```python
from build123d import *

# Parameters (mm, degrees)
BOSS_EXTRUDE2_DEPTH = 40
SKETCH3_4_R         = 2
SKETCH3_4_R_2       = 1
BOSS_EXTRUDE3_DEPTH = 10
BOSS_EXTRUDE4_START = -20
SKETCH3_5_R         = 2
SKETCH3_5_R_2       = 1
BOSS_EXTRUDE4_DEPTH = 10
SKETCH5_R           = 2
CUT_EXTRUDE1_DEPTH  = 10
FILLET1_R           = 3
FILLET2_R           = 3


with BuildPart() as part:
    # Sketch3 → Boss-Extrude2 (new body)
    with BuildSketch(Plane.XY):
        with BuildLine():
            Line((14.107916892, 0), (14.107916892, 1))
            Line((14.107916892, 1), (-5.892083108, 1))
            ThreePointArc((-5.892083108, 1), (-5.863018057, 0.804975408), (-5.853298215, 0.608036602))
            ThreePointArc((-5.853298215, 0.608036602), (-5.877106832, 0.300355571), (-5.947965831, 0))
            Line((-5.947965831, 0), (14.107916892, 0))
        make_face()
    extrude(amount=-BOSS_EXTRUDE2_DEPTH)

    # Sketch3_4 → Boss-Extrude3 (add)
    with BuildSketch(Plane.XY):
        with Locations((-7.853298215, 0.608036602)):
            Circle(SKETCH3_4_R)
        with Locations((-7.853298215, 0.608036602)):
            Circle(SKETCH3_4_R_2, mode=Mode.SUBTRACT)
    extrude(amount=-BOSS_EXTRUDE3_DEPTH)

    # Sketch3_5 → Boss-Extrude4 (add)
    with BuildSketch(Plane.XY.offset(BOSS_EXTRUDE4_START)):
        with Locations((-7.853298215, 0.608036602)):
            Circle(SKETCH3_5_R)
        with Locations((-7.853298215, 0.608036602)):
            Circle(SKETCH3_5_R_2, mode=Mode.SUBTRACT)
    extrude(amount=-BOSS_EXTRUDE4_DEPTH)

    # Sketch5 → Cut-Extrude1 (cut)
    with BuildSketch(Plane(origin=(0, 1, 0), x_dir=(1, 0, 0), z_dir=(0, 1, 0))):
        with Locations((-0.892083108, 30)):
            Circle(SKETCH5_R)
        with Locations((-0.892083108, 10)):
            Circle(SKETCH5_R)
        with Locations((9.107916892, 20)):
            Circle(SKETCH5_R)
    extrude(amount=-CUT_EXTRUDE1_DEPTH, mode=Mode.SUBTRACT)

    # Fillet1
    fillet1_edges = [part.edges().sort_by_distance(p)[0] for p in [
        (14.107916892, 0.5, -40),
    ]]
    fillet(fillet1_edges, radius=FILLET1_R)

    # Fillet2
    fillet2_edges = [part.edges().sort_by_distance(p)[0] for p in [
        (14.107916892, 0.5, 0),
    ]]
    fillet(fillet2_edges, radius=FILLET2_R)


solid = part.part
```
Geometry check sheet. Reference: the model listing, model coordinates, mm. A direction names the side the tool comes from. Coordinates: 2 decimals unless noted, no trailing zeros. Loops run counter-clockwise (first coordinate to the right, second up) from the corner with the lowest first, then second, coordinate; pieces in that order, holes last. Notation, with made-up numbers: (31, 81) - (74, 81) arc R7 ccw to (74, 92) - close; hole circle Ø3 at (-3.75, 88.25). An arc over 180 degrees is marked (long way). One line per item, written item: value. Start each with the question number.
(1) Mould release check, pull along Z, two halves, no side actions. Record for faces 1 (the flat face through (-7, 2, -10)), 2 (the cylindrical face through (13.25, 0.51, -0.9)), 3 (the flat face through (2.5, 0.5, -40)): released by +Z, released by -Z, zero draft, split by the parting line, or undercut.
(2) Tool access check on faces 4 (the flat face through (4, 1, -20)), 5 (the flat face through (-1, 0.5, 0)), 6 (the flat face through (4, 0, -20)). Record the directions out of +Z, -Z, +X, -X, +Y, -Y that give a thin tool (end or side, any length) a straight path to the whole face; none if there is none.
(3) Cross-section at B-B on y = 2. Enter the section's corners in (x, z).
(4) Cross-section at A-A on z = -29. Enter the section's corners in (x, y), plus the area to 3 significant figures.
(5) Depth check by flat-ended pin: P1, Ø6, axis at x = -1.5, z = -9.5, coming from the +Y side; P2, Ø1.5, axis at y = 1, z = -15, coming from the -X side; P3, Ø10, axis at x = 3, z = -24, coming from the -Y side; P4, Ø3, axis at x = -0.89, z = -10, coming from the -Y side. Enter the tip coordinate at first touch or a pass-through.
(6) Material ranges on line 1 (Z direction, x = -7, y = 1.2); line 2 (Y direction, x = -4.5, z = -6); line 3 (X direction, y = 0.45, z = -14), recorded low to high. Write a range as [from, to].
(7) Cross-section at C-C on z = -24. Enter the section's corners in (x, y), plus the area to 3 significant figures.
(8) Cross-section at D-D on z = -33. Enter the section's corners in (x, y).
Results below:
1. face 1: undercut
1. face 2: released by +Z
1. face 3: released by -Z
2. face 4: +Z, -Z, +X, +Y
2. face 5: +Z, +X, -X, +Y, -Y
2. face 6: +Z, -Z, +X, -Y
3. outline: (-9.29, -30) - (-6.42, -30) - (-6.42, -20) - (-9.29, -20) - close; (-9.29, -10) - (-6.42, -10) - (-6.42, 0) - (-9.29, 0) - close
4. outline: (-5.95, 0) - (-2.62, 0) - (-2.62, 1) - (-5.89, 1) arc R2 ccw (long way) to start; (0.84, 0) - (14.11, 0) - (14.11, 1) - (0.84, 1) - close; hole circle Ø2 at (-7.85, 0.61)
4. area: 25.9 mm2
5. P1: stops at y = 1
5. P2: stops at x = -5.89
5. P3: stops at y = 0
5. P4: passes through
6. line 1: z = [-30, -20], [-10, 0]
6. line 2: y = [0, 1]
6. line 3: x = [-5.86, 14.11]
7. outline: (-5.95, 0) - (14.11, 0) - (14.11, 1) - (-5.89, 1) arc R2 ccw (long way) to start; hole circle Ø2 at (-7.85, 0.61)
7. area: 29.4 mm2
8. outline: (-5.95, 0) - (14.11, 0) - (14.11, 1) - (-5.89, 1) arc R2 cw to start
